from build123d import *

# Parameters (mm, degrees)
ESQUISSE1_R        = 1.6
BOSS_EXTRU_1_DEPTH = 5


with BuildPart() as part:
    # Esquisse1 → Boss.-Extru.1 (new body)
    with BuildSketch(Plane(origin=(0, 0, 0), x_dir=(-1, 0, 0), z_dir=(0, 0, -1))):
        with BuildLine():
            Line((-13.228382526, 52.300004127), (-45.071523458, 52.300004127))
            ThreePointArc((-45.071523458, 52.300004127), (-45.836893076, 52.147762644), (-46.485742108, 51.714215582))
            Line((-46.485742108, 51.714215582), (-49.714164045, 48.485793645))
            ThreePointArc((-49.714164045, 48.485793645), (-50.147712239, 47.836942919), (-50.299954119, 47.071571303))
            Line((-50.299954119, 47.071571303), (-50.299954119, 42.65))
            Line((-50.299954119, 42.65), (-29.210001453, 42.65))
            ThreePointArc((-29.210001453, 42.65), (-17.71, 31.15), (-29.210001453, 19.65))
            Line((-29.210001453, 19.65), (-48.299953866, 19.65))
            ThreePointArc((-48.299953866, 19.65), (-49.714167607, 19.064213488), (-50.299954119, 17.649999747))
            Line((-50.299954119, 17.649999747), (-50.299954119, 10.499998844))
            ThreePointArc((-50.299954119, 10.499998844), (-50.153507491, 10.146445408), (-49.799954056, 9.99999878))
            Line((-49.799954056, 9.99999878), (-46.899953689, 9.99999878))
            Line((-46.899953689, 9.99999878), (-46.866453685, 10.124998796))
            Line((-46.866453685, 10.124998796), (-46.774953673, 10.216508808))
            Line((-46.774953673, 10.216508808), (-46.649953658, 10.249998812))
            Line((-46.649953658, 10.249998812), (-46.524953642, 10.216508808))
            Line((-46.524953642, 10.216508808), (-46.43344363, 10.124998796))
            Line((-46.43344363, 10.124998796), (-46.399953626, 9.99999878))
            Line((-46.399953626, 9.99999878), (-46.43344363, 9.874998765))
            Line((-46.43344363, 9.874998765), (-46.524953642, 9.783491753))
            Line((-46.524953642, 9.783491753), (-46.649953658, 9.749998749))
            Line((-46.649953658, 9.749998749), (-46.649953658, 0.49999758))
            ThreePointArc((-46.649953658, 0.49999758), (-46.50350703, 0.146444144), (-46.149953594, -2.484e-06))
            Line((-46.149953594, -2.484e-06), (-40.149952936, -2.484e-06))
            ThreePointArc((-40.149952936, -2.484e-06), (-39.79639943, 0.146444174), (-39.649952773, 0.49999768))
            Line((-39.649952773, 0.49999768), (-39.649952773, 9.749998749))
            Line((-39.649952773, 9.749998749), (-39.774952789, 9.783491753))
            Line((-39.774952789, 9.783491753), (-39.8664628, 9.874998765))
            Line((-39.8664628, 9.874998765), (-39.899952805, 9.99999878))
            Line((-39.899952805, 9.99999878), (-39.8664628, 10.124998796))
            Line((-39.8664628, 10.124998796), (-39.774952789, 10.216508808))
            Line((-39.774952789, 10.216508808), (-39.649952773, 10.249998812))
            Line((-39.649952773, 10.249998812), (-39.524952757, 10.216508808))
            Line((-39.524952757, 10.216508808), (-39.433442746, 10.124998796))
            Line((-39.433442746, 10.124998796), (-39.399952741, 9.99999878))
            Line((-39.399952741, 9.99999878), (-18.89995015, 9.99999878))
            Line((-18.89995015, 9.99999878), (-18.866450146, 10.124998796))
            Line((-18.866450146, 10.124998796), (-18.774950135, 10.216508808))
            Line((-18.774950135, 10.216508808), (-18.649950119, 10.249998812))
            Line((-18.649950119, 10.249998812), (-18.524950103, 10.216508808))
            Line((-18.524950103, 10.216508808), (-18.433440091, 10.124998796))
            Line((-18.433440091, 10.124998796), (-18.399950087, 9.99999878))
            Line((-18.399950087, 9.99999878), (-18.433440091, 9.874998765))
            Line((-18.433440091, 9.874998765), (-18.524950103, 9.783491753))
            Line((-18.524950103, 9.783491753), (-18.649950119, 9.749998749))
            Line((-18.649950119, 9.749998749), (-18.649950119, 0.49999758))
            ThreePointArc((-18.649950119, 0.49999758), (-18.503503491, 0.146444144), (-18.149950056, -2.484e-06))
            Line((-18.149950056, -2.484e-06), (-12.149949397, -2.484e-06))
            ThreePointArc((-12.149949397, -2.484e-06), (-11.796395891, 0.146444174), (-11.649949234, 0.49999768))
            Line((-11.649949234, 0.49999768), (-11.649949234, 9.749998749))
            Line((-11.649949234, 9.749998749), (-11.77494925, 9.783491753))
            Line((-11.77494925, 9.783491753), (-11.866459261, 9.874998765))
            Line((-11.866459261, 9.874998765), (-11.899949266, 9.99999878))
            Line((-11.899949266, 9.99999878), (-11.866459261, 10.124998796))
            Line((-11.866459261, 10.124998796), (-11.77494925, 10.216508808))
            Line((-11.77494925, 10.216508808), (-11.649949234, 10.249998812))
            Line((-11.649949234, 10.249998812), (-11.524949218, 10.216508808))
            Line((-11.524949218, 10.216508808), (-11.433439207, 10.124998796))
            Line((-11.433439207, 10.124998796), (-11.399949202, 9.99999878))
            Line((-11.399949202, 9.99999878), (-0.499947825, 9.99999878))
            ThreePointArc((-0.499947825, 9.99999878), (-0.14639439, 10.146445408), (5.2238e-05, 10.499998844))
            Line((5.2238e-05, 10.499998844), (5.2238e-05, 15.499999475))
            ThreePointArc((5.2238e-05, 15.499999475), (-0.14639439, 15.853552911), (-0.499947825, 15.999999539))
            Line((-0.499947825, 15.999999539), (-7.49994871, 15.999999539))
            ThreePointArc((-7.49994871, 15.999999539), (-7.853502145, 16.146446167), (-7.999948773, 16.499999602))
            Line((-7.999948773, 16.499999602), (-7.999948773, 47.071573466))
            ThreePointArc((-7.999948773, 47.071573466), (-8.152190984, 47.836946285), (-8.585740096, 48.485797894))
            Line((-8.585740096, 48.485797894), (-11.814159255, 51.714214053))
            ThreePointArc((-11.814159255, 51.714214053), (-12.46301048, 52.147762254), (-13.228382526, 52.300004127))
        make_face()
        with Locations((-13.61, 46.65)):
            Circle(ESQUISSE1_R, mode=Mode.SUBTRACT)
        with Locations((-13.61, 15.65)):
            Circle(ESQUISSE1_R, mode=Mode.SUBTRACT)
        Polygon((-22.025002784, 14.216511797), (-21.933492772, 14.125001785), (-21.900002768, 14.000001769), (-21.933492772, 13.875001754), (-22.025002784, 13.783491742), (-22.1500028, 13.750001738), (-22.275002815, 13.783491742), (-22.366502827, 13.875001754), (-22.400002831, 14.000001769), (-26.9000034, 14.000001769), (-26.933493404, 13.875001754), (-27.025003416, 13.783491742), (-27.150003431, 13.750001738), (-27.275003447, 13.783491742), (-27.366513459, 13.875001754), (-27.400003463, 14.000001769), (-27.366513459, 14.125001785), (-27.275003447, 14.216511797), (-27.150003431, 14.250001801), (-27.150003431, 16.250002054), (-27.275003447, 16.283492058), (-27.366513459, 16.37500207), (-27.400003463, 16.500002085), (-27.366513459, 16.625002101), (-27.275003447, 16.716512113), (-27.150003431, 16.750002117), (-27.025003416, 16.716512113), (-26.933493404, 16.625002101), (-26.9000034, 16.500002085), (-22.400002831, 16.500002085), (-22.366502827, 16.625002101), (-22.275002815, 16.716512113), (-22.1500028, 16.750002117), (-22.025002784, 16.716512113), (-21.933492772, 16.625002101), (-21.900002768, 16.500002085), (-21.933492772, 16.37500207), (-22.025002784, 16.283492058), (-22.1500028, 16.250002054), (-22.1500028, 14.250001801), align=None, mode=Mode.SUBTRACT)
        Polygon((-43.062295443, 18.400002326), (-41.474585242, 15.650001978), (-43.062295443, 12.90000163), (-46.237715844, 12.90000163), (-47.825426045, 15.650001978), (-46.237715844, 18.400002326), align=None, mode=Mode.SUBTRACT)
    extrude(amount=-BOSS_EXTRU_1_DEPTH)


solid = part.part
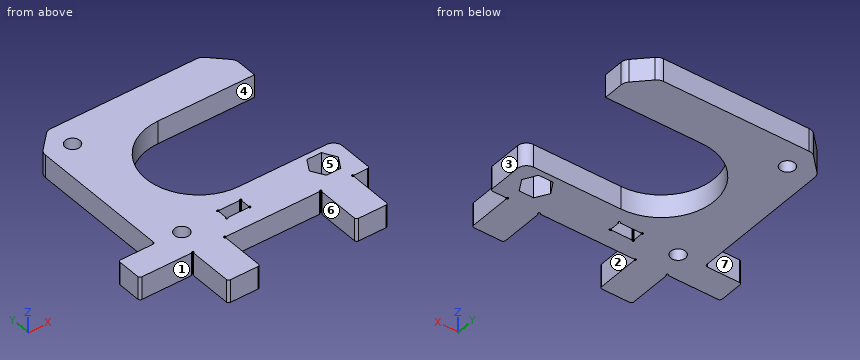
Geometry check sheet. Reference: the model listing, model coordinates, mm. Face numbers are marked on the shaded views. A direction names the side the tool comes from. Round coordinates to 2 decimals unless told otherwise and drop trailing zeros. Loops run counter-clockwise (first coordinate to the right, second up) from the corner with the lowest first, then second, coordinate; pieces in that order, holes last. Notation, with made-up numbers: (28.25, -24) -> (71.25, -24) arc R14 ccw to (71.25, -3) -> close; hole circle Ø7 at (58.5, -23.75). An arc over 180 degrees is marked (long way). Answer as a JSON object with one key per item and string values. Group by question number.
Item 1: Cross-section at B-B, the plane y = 4. Record the cut outline in (x, z), plus the area to 3 significant figures.
Item 2: Cross-section at A-A, the plane x = 30. Record the cut outline in (y, z), plus the area to 3 significant figures.
Item 3: Cross-section at C-C, the plane z = 2.35. Count the separate pieces of the cut face and the enclosed holes in it, plus the area to 3 significant figures.
Item 4: Thickness scan on line 1 along Y through (x, z) = (13.61, 3.75); line 2 along Y through (x, z) = (34, 1.9); line 3 along Y through (x, z) = (24, 4). Record the ranges inside material, lowest first.
Item 5: Set-up check for the marked faces 4, 5, 6 and 7: record each of +Z, -Z, +X, -X, +Y, -Y from which the full face is reachable in a straight line by a thin tool's end or side.
Item 6: Cross-section at D-D, the plane y = 34.5. Record the cut outline in (x, z), plus the area to 3 significant figures.
Item 7: Release check for a two-part mould opening along X. For the marked faces 1, 2 and 3 record: pulls with the +X half, pulls with the -X half, needs draft (parallel to the pull), parting line crosses it, or undercut.
Item 8: Depth check by flat-ended pin: pin 1 Ø1.5 at (x, z) = (5, 2) entering from -Y; pin 2 Ø4 at (x, y) = (17, 26.5) entering from -Z; pin 3 Ø1.5 at (x, z) = (3.5, 2.5) entering from +Y. Enter the tip coordinate at first touch or a pass-through.
Determined:
{
 "1": {"outline": "(11.65, 0) -> (18.65, 0) -> (18.65, 5) -> (11.65, 5) -> close; (39.65, 0) -> (46.65, 0) -> (46.65, 5) -> (39.65, 5) -> close", "area": "70.0 mm²"},
 "2": {"outline": "(10, 0) -> (19.65, 0) -> (19.65, 5) -> (10, 5) -> close; (42.65, 0) -> (52.3, 0) -> (52.3, 5) -> (42.65, 5) -> close", "area": "96.5 mm²"},
 "3": {"separate pieces": "1", "enclosed holes": "4", "area": "1,210 mm²"},
 "4": {"line 1": "y = 0 to 14.05, 17.25 to 45.05, 48.25 to 52.3", "line 2": "y = 10 to 19.65, 42.65 to 52.3", "line 3": "y = 10 to 14, 16.5 to 20.9, 41.4 to 52.3"},
 "5": {"face 4": "+Z, -Z, +X", "face 5": "+Z, -Z", "face 6": "+Z, -Z, -Y", "face 7": "+Z, -Z, -X, +Y"},
 "6": {"outline": "(8, 0) -> (18.21, 0) -> (18.21, 5) -> (8, 5) -> close", "area": "51.0 mm²"},
 "7": {"face 1": "needs draft", "face 2": "undercut", "face 3": "pulls with the +X half"},
 "8": {"pin 1": "stops at y = 10", "pin 2": "stops at z = 0", "pin 3": "stops at y = 16"}
}
